The model under review builds one solid part; all positions refer to its coordinate system, in mm. Face numbers are marked on the shaded views. Give positions to 0.01 mm unless a question says otherwise; leave off trailing zeros. Order: outer loops, then holes, each group sorted by start corner. A loop starts at its lowest first (then second) coordinate and runs counter-clockwise, first axis right, second up.
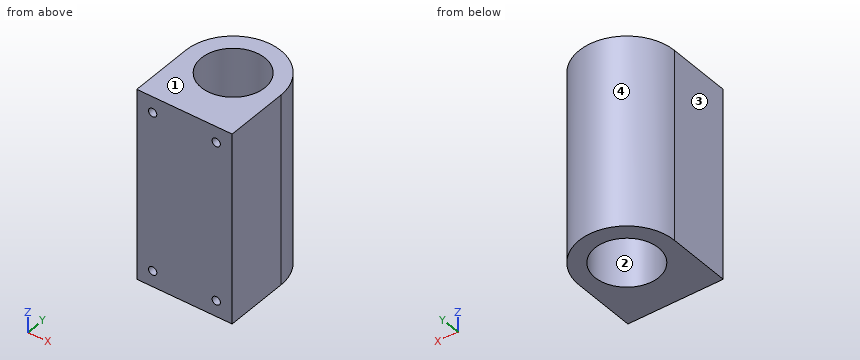
```python
from build123d import *

# Parameters (mm, degrees)
F1_DEPTH = 38.1
F2_R     = 1.651
F3_DEPTH = 12.7


with BuildPart() as f1:
    # F0 (on Top) → F1 (new body, symmetric)
    with BuildSketch(Plane.XY):
        with BuildLine():
            Line((12.7, 0), (19.05, 0))
            ThreePointArc((19.05, 0), (0, 19.05), (-19.05, 0))
            Line((-19.05, 0), (-12.7, 0))
            ThreePointArc((-12.7, 0), (0, 12.7), (12.7, 0))
        make_face()
        with BuildLine():
            Line((19.05, -25.4), (19.05, 0))
            ThreePointArc((19.05, 0), (0, -19.05), (-19.05, 0))
            Line((-19.05, 0), (-19.05, -25.4))
            Line((-19.05, -25.4), (19.05, -25.4))
        make_face()
        with BuildLine():
            ThreePointArc((-19.05, 0), (0, -19.05), (19.05, 0))
            Line((19.05, 0), (12.7, 0))
            ThreePointArc((12.7, 0), (0, -12.7), (-12.7, 0))
            Line((-12.7, 0), (-19.05, 0))
        make_face()
    extrude(amount=F1_DEPTH, both=True)

    # F2 (on face) → F3 (cut)
    with BuildSketch(Plane.XZ.offset(25.4)):
        with Locations((12.7, 31.75)):
            Circle(F2_R)
        with Locations((-12.7, 31.75)):
            Circle(F2_R)
        with Locations((-12.7, -31.75)):
            Circle(F2_R)
        with Locations((12.7, -31.75)):
            Circle(F2_R)
    extrude(amount=-F3_DEPTH, mode=Mode.SUBTRACT)


solid = f1.part
```
1. Take a section at A-A (x = 0). Write out the cut boundary in (y, z).
2. Take a section at D-D (z = -7). Write out the cut boundary in (x, y), and give its area (3 significant figures).
3. Draft analysis for pull direction X (two halves, no side actions). For the marked faces 1, 2, 3 and 4, state which applies: pulls with the +X half, pulls with the -X half, needs draft (parallel to the pull), parting line crosses it, or undercut.
4. Take a section at B-B (z = 31.75). Write out the cut boundary in (x, y).
5. Insertion check: pin 1 (1 mm diameter, centred on x = -13, z = -31, fed in from -Y); pin 2 (5 mm diameter, centred on y = 8, z = 10.5, fed in from -X); pin 3 (2 mm diameter, centred on x = -7.5, z = 30, fed in from +Y); pin 4 (15 mm diameter, centred on x = 0, y = 0, fed in from +Z). Each pin has a flat end and moves straight along its axis. Give the tip position at first contact, or say it passes through.
6. To check wall thickness, follow line 1 (Z direction, x = 12.7, y = -20); line 2 (X direction, y = 0.5, z = -35); line 3 (X direction, y = -15, z = 32.5). State the ranges of each line that lie inside material, in increasing order.
7. Take a section at C-C (y = 5). Write out the cut boundary in (x, z), and give its area (3 significant figures).
Answer:
1. outline: (-25.4, -38.1) - (-12.7, -38.1) - (-12.7, 38.1) - (-25.4, 38.1) - close; (12.7, -38.1) - (19.05, -38.1) - (19.05, 38.1) - (12.7, 38.1) - close
2. outline: (-19.05, -25.4) - (19.05, -25.4) - (19.05, 0) arc R19.05 ccw to (-19.05, 0) - close; hole circle Ø25.4 at (0, 0)
2. area: 1,030 mm2
3. face 1: needs draft
3. face 2: undercut
3. face 3: pulls with the -X half
3. face 4: parting line crosses it
4. outline: (-19.05, -25.4) - (-14.35, -25.4) - (-14.35, -12.7) - (-11.05, -12.7) - (-11.05, -25.4) - (11.05, -25.4) - (11.05, -12.7) - (14.35, -12.7) - (14.35, -25.4) - (19.05, -25.4) - (19.05, 0) arc R19.05 ccw to (-19.05, 0) - close; hole circle Ø25.4 at (0, 0)
5. pin 1: stops at y = -12.7
5. pin 2: stops at x = -18.24
5. pin 3: stops at y = 17.91
5. pin 4: passes through
6. line 1: z = -38.1 to -33.4, -30.1 to 30.1, 33.4 to 38.1
6. line 2: x = -19.04 to -12.69, 12.69 to 19.04
6. line 3: x = -19.05 to -14.17, -11.23 to 11.23, 14.17 to 19.05
7. outline: (-18.38, -38.1) - (-11.67, -38.1) - (-11.67, 38.1) - (-18.38, 38.1) - close; (11.67, -38.1) - (18.38, -38.1) - (18.38, 38.1) - (11.67, 38.1) - close
7. area: 1,020 mm2
